Design review of the part built by this model. Coordinates are the model's own, in mm. A direction names the side the tool comes from. Give positions to 0.01 mm unless a question says otherwise; leave off trailing zeros. Loops run counter-clockwise (first coordinate to the right, second up) from the corner with the lowest first, then second, coordinate; pieces in that order, holes last.
from build123d import *

# Parameters (mm, degrees)
BOSS_EXTRUDE1_DEPTH = 5.5
SKETCH2_R           = 3
BOSS_EXTRUDE2_DEPTH = 1.5
SKETCH3_R           = 1.35
CUT_EXTRUDE1_DEPTH  = 17.840471554
SKETCH4_R           = 3
BOSS_EXTRUDE3_DEPTH = 2
SKETCH5_R           = 1.35
CUT_EXTRUDE2_DEPTH  = 18.585311609
SKETCH6_R           = 11.75
CUT_EXTRUDE3_DEPTH  = 3.5
SKETCH7_R           = 4.625
CUT_EXTRUDE4_DEPTH  = 18.585311609
CUT_EXTRUDE5_DEPTH  = 3.5


with BuildPart() as part:
    # Sketch1 → Boss-Extrude1 (new body)
    with BuildSketch(Plane(origin=(65.356779706, -19.323104474, 0), x_dir=(-0.28352355, -0.958965274, 0), z_dir=(-0.958965274, 0.28352355, 0))):
        with BuildLine():
            Line((-22.409230804, 105.535335292), (-25.708238472, 109.248684924))
            ThreePointArc((-25.708238472, 109.248684924), (-28.941829317, 110.584612338), (-31.989317839, 108.866000829))
            ThreePointArc((-31.989317839, 108.866000829), (-39.5119826, 89.676955929), (-37.690186632, 69.146710224))
            ThreePointArc((-37.690186632, 69.146710224), (-34.240446028, 65.888665427), (-29.622491121, 66.979563497))
            Line((-29.622491121, 66.979563497), (-23.166630632, 72.715067926))
            ThreePointArc((-23.166630632, 72.715067926), (-19.824639339, 74.487704396), (-16.041831895, 74.526610749))
            ThreePointArc((-16.041831895, 74.526610749), (1.733883997, 88.181945854), (-15.123670288, 102.955811829))
            ThreePointArc((-15.123670288, 102.955811829), (-19.098619321, 103.307401938), (-22.409230804, 105.535335292))
        make_face()
    extrude(amount=-BOSS_EXTRUDE1_DEPTH)

    # Sketch2 → Boss-Extrude2 (add)
    with BuildSketch(Plane(origin=(70.631088713, -20.882483997, 0), x_dir=(0, 0, -1), z_dir=(0.958965274, -0.28352355, 0))):
        with Locations((-106.592015807, 28.69857444)):
            Circle(SKETCH2_R)
    extrude(amount=BOSS_EXTRUDE2_DEPTH)

    # Sketch3 → Cut-Extrude1 (cut, through all)
    with BuildSketch(Plane(origin=(65.356779706, -19.323104474, 0), x_dir=(0, 0, 1), z_dir=(-0.958965274, 0.28352355, 0))):
        with Locations((106.592015807, 28.69857444)):
            Circle(SKETCH3_R)
    extrude(amount=-CUT_EXTRUDE1_DEPTH, mode=Mode.SUBTRACT)

    # Sketch4 → Boss-Extrude3 (add)
    with BuildSketch(Plane(origin=(70.631088713, -20.882483997, 0), x_dir=(0, 0, -1), z_dir=(0.958965274, -0.28352355, 0))):
        with Locations((-70.717483457, 32.943327517)):
            Circle(SKETCH4_R)
    extrude(amount=BOSS_EXTRUDE3_DEPTH)

    # Sketch5 → Cut-Extrude2 (cut, through all)
    with BuildSketch(Plane(origin=(65.356779706, -19.323104474, 0), x_dir=(0, 0, 1), z_dir=(-0.958965274, 0.28352355, 0))):
        with Locations((70.717483457, 32.943327517)):
            Circle(SKETCH5_R)
    extrude(amount=-CUT_EXTRUDE2_DEPTH, mode=Mode.SUBTRACT)

    # Sketch6 → Cut-Extrude3 (cut)
    with BuildSketch(Plane(origin=(70.631088713, -20.882483997, 0), x_dir=(0, 0, -1), z_dir=(0.958965274, -0.28352355, 0))):
        with Locations((-88.65, 12.758559735)):
            Circle(SKETCH6_R)
    extrude(amount=-CUT_EXTRUDE3_DEPTH, mode=Mode.SUBTRACT)

    # Sketch7 → Cut-Extrude4 (cut, through all)
    with BuildSketch(Plane(origin=(65.356779706, -19.323104474, 0), x_dir=(0, 0, 1), z_dir=(-0.958965274, 0.28352355, 0))):
        with Locations((88.65, 12.758559735)):
            Circle(SKETCH7_R)
    extrude(amount=-CUT_EXTRUDE4_DEPTH, mode=Mode.SUBTRACT)

    # Sketch8 → Cut-Extrude5 (cut)
    with BuildSketch(Plane(origin=(70.631088713, -20.882483997, 0), x_dir=(0, 0, -1), z_dir=(0.958965274, -0.28352355, 0))):
        with BuildLine():
            Line((-74.584027906, 24.82704883), (-73.736581379, 25.780931199))
            ThreePointArc((-73.736581379, 25.780931199), (-73.240380162, 27.294869383), (-74.007814455, 28.691031651))
            ThreePointArc((-74.007814455, 28.691031651), (-75.840549655, 31.311613406), (-75.860990165, 34.509417221))
            ThreePointArc((-75.860990165, 34.509417221), (-76.089806816, 36.170205007), (-77.502198812, 37.073378292))
            ThreePointArc((-77.502198812, 37.073378292), (-89.36916003, 37.030513551), (-100.761658133, 33.708226249))
            ThreePointArc((-100.761658133, 33.708226249), (-101.817813371, 32.571238358), (-101.742925567, 31.021207013))
            ThreePointArc((-101.742925567, 31.021207013), (-101.4721051, 30.340162869), (-101.296421193, 29.628615248))
            ThreePointArc((-101.296421193, 29.628615248), (-100.31044829, 28.233312085), (-98.606486741, 28.10869859))
            ThreePointArc((-98.606486741, 28.10869859), (-87.819157421, 28.939652392), (-78.355573806, 23.695842402))
            ThreePointArc((-78.355573806, 23.695842402), (-76.768954569, 23.099003898), (-75.294048195, 23.934604274))
            ThreePointArc((-75.294048195, 23.934604274), (-74.951163338, 24.390473315), (-74.584027906, 24.82704883))
        make_face()
    extrude(amount=-CUT_EXTRUDE5_DEPTH, mode=Mode.SUBTRACT)


solid = part.part
Q1. Take a section at A-A (z = 70). Give the boundary of the cut face in (x, y) (3 decimals).
Results:
outline: (72.792, 5.824) - (78.066, 4.264) - (79.145, 7.916) - (81.063, 7.349) - (81.565, 9.045) - (74.373, 11.172) - close; (75.021, 13.365) - (82.213, 11.239) - (82.715, 12.935) - (80.797, 13.502) - (81.395, 15.523) - (76.12, 17.082) - close
Q2. Insertion check: pin 1 (2 mm diameter, centred on y = 4, z = 82.5, fed in from +X); pin 2 (2 mm diameter, centred on x = 76, z = 95, fed in from +Y); pin 3 (2 mm diameter, centred on y = 5.5, z = 105, fed in from +X). Each pin has a flat end and moves straight along its axis. Give the tip position at first contact, or say it passes through.
Results:
pin 1: stops at x = 78.28
pin 2: stops at y = 17.75
pin 3: stops at x = 80.29
Q3. Wall thickness on line 1 (Z direction, x = 70.5, y = -6); line 2 (X direction, y = 8, z = 82); line 3 (Z direction, x = 74, y = 6.5): over which ranges is each line inside the solid? List them lowest first.
Results:
line 1: z = 74.23 to 84.27, 93.03 to 103.07
line 2: x = 73.44 to 75.52
line 3: z = 69.12 to 110.31
Q4. Tool access review of faces 4 (the face through (76.341, 10.776, 87.786)), 5 (the face through (75.45, 5.26, 69.81)): name each direction out of +Z, -Z, +X, -X, +Y, -Y from which nothing blocks a thin tool from reaching the whole face with its end or side.
Results:
face 4: none
face 5: -Z, -X, -Y
Q5. Draft analysis for pull direction Y (two halves, no side actions). For faces 1 (the face through (72.173, 3.73, 88.469)), 2 (the face through (76.149, 3.866, 74.166)), 3 (the face through (74.77, 2.96, 107.37)), state which applies: pulls with the +Y half, pulls with the -Y half, needs draft (parallel to the pull), parting line crosses it, or undercut.
Results:
face 1: pulls with the +Y half
face 2: undercut
face 3: pulls with the -Y half
Q6. Take a section at B-B (z = 83). Give the boundary of the cut face in (x, y), plus the area to 3 significant figures.
Results:
outline: (65.19, -19.89) - (70.46, -21.45) - (71.33, -18.53) - (67.97, -17.53) - (73.81, 2.22) - (77.17, 1.23) - (78.34, 5.18) - (74.98, 6.17) - (77.9, 16.04) - (81.25, 15.05) - (81.96, 17.45) - (76.69, 19) - close
area: 115 mm2
